Can you work these out from the model? Positions are in its coordinate system, mm. Face numbers are marked on the shaded views. A direction names the side the tool comes from. Round coordinates to 2 decimals unless told otherwise and drop trailing zeros. Write each loop counter-clockwise with the first axis right and the second up, starting at its lowest first coordinate (ties: lowest second). Pieces come first, ordered by that corner, then holes. Notation, with made-up numbers: M -33.5,50 L 15.5,50 A32 cw 15.5,85 Z; hole C -8.75,26 d1. An arc over 180 degrees is marked long. Answer as a JSON object with one key per item and string values. Group by question number.
1) Suppose I cut it at D-D, the plane y = -4.75. Write out the boundary of the cut face in (x, z), and give its area (3 significant figures).
2) Please list where these lines run through material, in increasing order: L1, parallel to X at y = 6.5, z = 3.75; L2, parallel to Z at x = 2.5, y = 0; L3, parallel to Y at x = 5.5, z = 1. Write a range as [from, to].
3) If we mould it in two halves opening along X, with no side actions, what happens to the marked faces 1, 2, 3 and 4? For each: +X half, -X half, draft (parallel to the pull), parting line (faces both ways), or undercut.
4) Suppose I cut it at C-C, the plane x = 1.25. Write out the boundary of the cut face in (y, z), and give its area (3 significant figures).
5) On a 3-axis mill with a long thin cutter (end or side, diameter ignored), from which of +Z, -Z, +X, -X, +Y, -Y can I reach the whole of each face in a straight line? I mean the marked faces 5 and 6. Say none if no direction works.
6) I'm going to push flat-ended pins straight in: pin 1 Ø4 at (x, y) = (1.5, 3) entering from +Z; pin 2 Ø1.5 at (x, y) = (3, 2) entering from -Z. Where does each tip first touch, or does it pass through?
7) Suppose I cut it at A-A, the plane z = 0. Write out the boundary of the cut face in (x, y).
Autodesk Fusion 360 part; units mm, degrees
sketch "Sketch1" plane through (0, 0, 0) normal (1, 0, 0) x (0, 1, 0)
  circle A0 centre (0, 0) radius 6.11
  circle A1 centre (0, 0) radius 9
  circle A2 centre (0, 0) radius 1.5
  circle A3 centre (0, 0) radius 6.365 construction
  dimension "d1" = 3
  dimension "d2" = 12.22
  dimension "d3" = 18
  dimension "d11" = 12.73
extrude "Extrude1" add sketch "Sketch1" along normal blind 9 contours A0 | A1
extrude "Extrude2" cut sketch "Sketch1" along normal blind 7 from surface at 1 contours A1
equation "d2 = outside_dia"
equation "pitch_dia = 12.73 mm"
equation "outside_dia = 12.22 mm"
equation "d11 = pitch_dia"
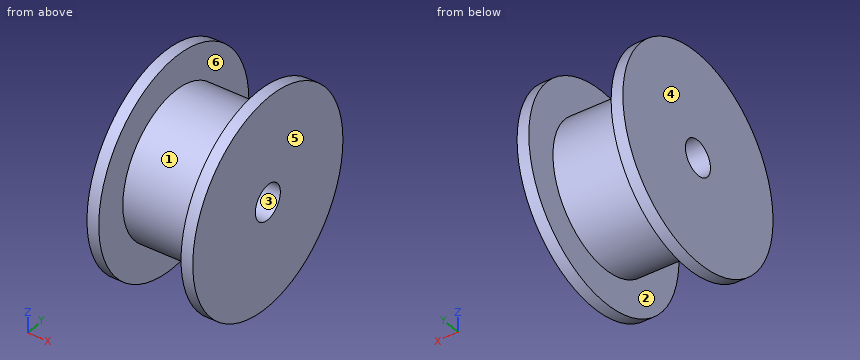
Results:
{
 "1": {"outline": "M 0,-7.64 L 1,-7.64 L 1,-3.84 L 8,-3.84 L 8,-7.64 L 9,-7.64 L 9,7.64 L 8,7.64 L 8,3.84 L 1,3.84 L 1,7.64 L 0,7.64 Z", "area": "84.4 mm^2"},
 "2": {"L1": "[0, 1], [8, 9]", "L2": "[-6.11, -1.5], [1.5, 6.11]", "L3": "[-6.03, -1.12], [1.12, 6.03]"},
 "3": {"face 1": "undercut", "face 2": "undercut", "face 3": "draft", "face 4": "-X half"},
 "4": {"outline": "C 0,0 d12.22; hole C 0,0 d3", "area": "110 mm^2"},
 "5": {"face 5": "+Z, -Z, +X, +Y, -Y", "face 6": "none"},
 "6": {"pin 1": "z = 8.94", "pin 2": "z = -5.98"},
 "7": {"outline": "M 0,-9 L 1,-9 L 1,-6.11 L 8,-6.11 L 8,-9 L 9,-9 L 9,-1.5 L 0,-1.5 Z; M 0,1.5 L 9,1.5 L 9,9 L 8,9 L 8,6.11 L 1,6.11 L 1,9 L 0,9 Z"}
}
